Read the model definition and answer for the solid it produces. Units are mm, in the model's axes. Face numbers are marked on the shaded views. A direction names the side the tool comes from. Coordinates: 2 decimals unless noted, no trailing zeros. Loops run counter-clockwise (first coordinate to the right, second up) from the corner with the lowest first, then second, coordinate; pieces in that order, holes last. Notation, with made-up numbers: M 16,74.5 L 35,74.5 A30 ccw 35,101.5 Z; hole C 9.25,64 d11. An arc over 180 degrees is marked long. Put each result on its own line as item: value.
from build123d import *

# Parameters (mm, degrees)
SKETCH1_W            = 150
SKETCH1_H            = 42
BOSS_EXTRUDE1_DEPTH  = 3.2
SKETCH2_W            = 162
SKETCH2_H            = 51
BOSS_EXTRUDE2_DEPTH  = 6
SKETCH3_W            = 6
SKETCH3_H            = 51
BOSS_EXTRUDE3_DEPTH  = 176
BOSS_EXTRUDE4_REACH  = 238.563
SKETCH5_W            = 51
SKETCH5_H            = 6
BOSS_EXTRUDE5_START  = 100
SKETCH1_2_W          = 150
SKETCH1_2_H          = 42
BOSS_EXTRUDE5_DEPTH  = 3.2
SKETCH6_W            = 150
SKETCH6_H            = 6
BOSS_EXTRUDE6_DEPTH  = 70
CUT_EXTRUDE1_REACH   = 142.553
SKETCH7_W            = 9.5
SKETCH7_H            = 39
SKETCH7_R            = 2.75
SKETCH7_3_W          = 6
SKETCH7_3_H          = 39
BOSS_EXTRUDE7_DEPTH  = 54
SKETCH8_W            = 162
SKETCH8_H            = 10
BOSS_EXTRUDE8_DEPTH  = 6
SKETCH9_W            = 150
SKETCH9_H            = 42
CUT_EXTRUDE2_DEPTH   = 3.2
CUT_EXTRUDE3_DEPTH   = 3.2
BOSS_EXTRUDE9_DEPTH  = 6
SKETCH12_W           = 6
SKETCH12_H           = 9.5
BOSS_EXTRUDE10_DEPTH = 6
CUT_EXTRUDE4_REACH   = 235.384
SKETCH13_R           = 4
CUT_EXTRUDE5_REACH   = 202.345
SKETCH14_R           = 1
SKETCH16_W           = 6
SKETCH16_H           = 172
BOSS_EXTRUDE11_DEPTH = 6
BOSS_EXTRUDE15_START = -51
BOSS_EXTRUDE15_DEPTH = 6
SKETCH17_W           = 162
SKETCH17_H           = 63
SKETCH17_W_2         = 150
SKETCH17_H_2         = 56.6
BOSS_EXTRUDE12_DEPTH = 6
SKETCH15_R           = 1
BOSS_EXTRUDE14_DEPTH = 6
FILLET1_R            = 2
FILLET1_OF_MIRROR4_R = 2


with BuildPart() as part:
    # Sketch1 → Boss-Extrude1 (new body)
    with BuildSketch(Plane(origin=(0, 0, 0), x_dir=(1, 0, 0), z_dir=(0, 1, 0))):
        Rectangle(SKETCH1_W, SKETCH1_H)
    extrude(amount=BOSS_EXTRUDE1_DEPTH)

    # Sketch2 → Boss-Extrude2 (add)
    with BuildSketch(Plane.XZ):
        Rectangle(SKETCH2_W, SKETCH2_H)
    extrude(amount=BOSS_EXTRUDE2_DEPTH)

    # Sketch3 → Boss-Extrude3 (add)
    with BuildSketch(Plane(origin=(0, 0, 0), x_dir=(1, 0, 0), z_dir=(0, 1, 0))):
        with Locations((78, 0)):
            Rectangle(SKETCH3_W, SKETCH3_H)
        with Locations((-78, 0)):
            Rectangle(SKETCH3_W, SKETCH3_H)
    extrude(amount=BOSS_EXTRUDE3_DEPTH)

    # Sketch5 → Boss-Extrude4 (add, up to next)
    with BuildSketch(Plane.ZY.offset(-75), mode=Mode.PRIVATE) as boss_extrude4_sk1:
        with Locations((0, 103)):
            Rectangle(SKETCH5_W, SKETCH5_H)
    boss_extrude4_tool1 = extrude(boss_extrude4_sk1.sketch, amount=BOSS_EXTRUDE4_REACH, mode=Mode.PRIVATE) - part.part
    add(boss_extrude4_tool1.solids().sort_by_distance((75, 103, 0))[0])

    # Sketch1<2> → Boss-Extrude5 (add)
    with BuildSketch(Plane(origin=(0, 0, 0), x_dir=(1, 0, 0), z_dir=(0, 1, 0)).offset(BOSS_EXTRUDE5_START)):
        Rectangle(SKETCH1_2_W, SKETCH1_2_H)
    extrude(amount=-BOSS_EXTRUDE5_DEPTH)

    # Sketch6 → Boss-Extrude6 (add)
    with BuildSketch(Plane(origin=(0, 106, 0), x_dir=(1, 0, 0), z_dir=(0, 1, 0))):
        with Locations((0, -22.5)):
            Rectangle(SKETCH6_W, SKETCH6_H)
        with Locations((0, 22.5)):
            Rectangle(SKETCH6_W, SKETCH6_H)
    extrude(amount=BOSS_EXTRUDE6_DEPTH)

    # Sketch7 → Cut-Extrude1 (cut, up to next)
    with BuildSketch(Plane(origin=(0, 106, 0), x_dir=(1, 0, 0), z_dir=(0, 1, 0)), mode=Mode.PRIVATE) as cut_extrude1_sk1:
        with Locations((70.25, 0)):
            Rectangle(SKETCH7_W, SKETCH7_H)
        with Locations((70.25, -14.75)):
            Circle(SKETCH7_R, mode=Mode.SUBTRACT)
        with Locations((70.25, 14.75)):
            Circle(SKETCH7_R, mode=Mode.SUBTRACT)
    cut_extrude1_tool1 = extrude(cut_extrude1_sk1.sketch, amount=-CUT_EXTRUDE1_REACH, mode=Mode.PRIVATE) & part.part
    # Sketch7 → Cut-Extrude1 (cut, up to next)
    with BuildSketch(Plane(origin=(0, 106, 0), x_dir=(1, 0, 0), z_dir=(0, 1, 0)), mode=Mode.PRIVATE) as cut_extrude1_sk2:
        with Locations((70.25, -14.75)):
            Circle(SKETCH7_R)
    cut_extrude1_tool2 = extrude(cut_extrude1_sk2.sketch, amount=-CUT_EXTRUDE1_REACH, mode=Mode.PRIVATE) & part.part
    # Sketch7 → Cut-Extrude1 (cut, up to next)
    with BuildSketch(Plane(origin=(0, 106, 0), x_dir=(1, 0, 0), z_dir=(0, 1, 0)), mode=Mode.PRIVATE) as cut_extrude1_sk3:
        with Locations((70.25, 14.75)):
            Circle(SKETCH7_R)
    cut_extrude1_tool3 = extrude(cut_extrude1_sk3.sketch, amount=-CUT_EXTRUDE1_REACH, mode=Mode.PRIVATE) & part.part
    add(cut_extrude1_tool1.solids().sort_by_distance((70.25, 106, 0))[0], mode=Mode.SUBTRACT)
    add(cut_extrude1_tool2.solids().sort_by_distance((70.25, 106, 14.75))[0], mode=Mode.SUBTRACT)
    add(cut_extrude1_tool3.solids().sort_by_distance((70.25, 106, -14.75))[0], mode=Mode.SUBTRACT)

    # Sketch7<3> → Boss-Extrude7 (add)
    with BuildSketch(Plane(origin=(0, 106, 0), x_dir=(1, 0, 0), z_dir=(0, 1, 0))):
        with Locations((62.5, 0)):
            Rectangle(SKETCH7_3_W, SKETCH7_3_H)
    extrude(amount=BOSS_EXTRUDE7_DEPTH)

    # Sketch8 → Boss-Extrude8 (add)
    with BuildSketch(Plane(origin=(0, 0, -25.5), x_dir=(-1, 0, 0), z_dir=(0, 0, -1))):
        with Locations((0, -1)):
            Rectangle(SKETCH8_W, SKETCH8_H)
    boss_extrude8 = extrude(amount=BOSS_EXTRUDE8_DEPTH)

    # Mirror1: Boss-Extrude8 across plane
    add(boss_extrude8.mirror(Plane.XY))

    # Sketch9 → Cut-Extrude2 (cut)
    with BuildSketch(Plane(origin=(0, 3.2, 0), x_dir=(1, 0, 0), z_dir=(0, 1, 0))):
        Rectangle(SKETCH9_W, SKETCH9_H)
    extrude(amount=-CUT_EXTRUDE2_DEPTH, mode=Mode.SUBTRACT)

    # Sketch10 → Cut-Extrude3 (cut)
    with BuildSketch(Plane.XZ.offset(-96.8)):
        Polygon((-75, -21), (75, -21), (75, -19.5), (65.5, -19.5), (65.5, 19.5), (75, 19.5), (75, 21), (-75, 21), align=None)
    extrude(amount=-CUT_EXTRUDE3_DEPTH, mode=Mode.SUBTRACT)

    # Sketch11 → Boss-Extrude9 (add)
    with BuildSketch(Plane.ZY.offset(-75)):
        Polygon((10, 93.5), (-21, 93.5), (-21, 0), (21, 0), (21, 100), (10, 100), align=None)
    boss_extrude9 = extrude(amount=BOSS_EXTRUDE9_DEPTH)

    # Mirror2: Boss-Extrude9 across plane
    add(boss_extrude9.mirror(Plane(origin=(0, 0, 0), x_dir=(0, 0, 1), z_dir=(1, 0, 0))))

    # Sketch12 → Boss-Extrude10 (add)
    with BuildSketch(Plane(origin=(0, 100, 0), x_dir=(1, 0, 0), z_dir=(0, 1, 0))):
        with Locations((72, -14.75)):
            Rectangle(SKETCH12_W, SKETCH12_H)
    extrude(amount=BOSS_EXTRUDE10_DEPTH)

    # Sketch13 → Cut-Extrude4 (cut, up to next)
    with BuildSketch(Plane.ZY.offset(-69), mode=Mode.PRIVATE) as cut_extrude4_sk1:
        with Locations((0, 20)):
            Circle(SKETCH13_R)
    cut_extrude4_tool1 = extrude(cut_extrude4_sk1.sketch, amount=-CUT_EXTRUDE4_REACH, mode=Mode.PRIVATE) & part.part
    add(cut_extrude4_tool1.solids().sort_by_distance((69, 20, 0))[0], mode=Mode.SUBTRACT)

    # Sketch14 → Cut-Extrude5 (cut, up to next)
    with BuildSketch(Plane.XY.offset(-19.5), mode=Mode.PRIVATE) as cut_extrude5_sk1:
        with Locations((62.5, 103)):
            Circle(SKETCH14_R)
    cut_extrude5_tool1 = extrude(cut_extrude5_sk1.sketch, amount=-CUT_EXTRUDE5_REACH, mode=Mode.PRIVATE) & part.part
    # Sketch14 → Cut-Extrude5 (cut, up to next)
    with BuildSketch(Plane.XY.offset(-19.5), mode=Mode.PRIVATE) as cut_extrude5_sk2:
        with Locations((62.5, 109)):
            Circle(SKETCH14_R)
    cut_extrude5_tool2 = extrude(cut_extrude5_sk2.sketch, amount=-CUT_EXTRUDE5_REACH, mode=Mode.PRIVATE) & part.part
    # Sketch14 → Cut-Extrude5 (cut, up to next)
    with BuildSketch(Plane.XY.offset(-19.5), mode=Mode.PRIVATE) as cut_extrude5_sk3:
        with Locations((62.5, 115)):
            Circle(SKETCH14_R)
    cut_extrude5_tool3 = extrude(cut_extrude5_sk3.sketch, amount=-CUT_EXTRUDE5_REACH, mode=Mode.PRIVATE) & part.part
    add(cut_extrude5_tool1.solids().sort_by_distance((62.5, 103, -19.5))[0], mode=Mode.SUBTRACT)
    add(cut_extrude5_tool2.solids().sort_by_distance((62.5, 109, -19.5))[0], mode=Mode.SUBTRACT)
    add(cut_extrude5_tool3.solids().sort_by_distance((62.5, 115, -19.5))[0], mode=Mode.SUBTRACT)

    # Sketch16 → Boss-Extrude11 (add)
    with BuildSketch(Plane(origin=(0, 0, -25.5), x_dir=(-1, 0, 0), z_dir=(0, 0, -1))):
        with Locations((78, 90)):
            Rectangle(SKETCH16_W, SKETCH16_H)
        with Locations((-78, 90)):
            Rectangle(SKETCH16_W, SKETCH16_H)
    extrude(amount=BOSS_EXTRUDE11_DEPTH)

    # Sketch16<2> → Boss-Extrude15 (add)
    with BuildSketch(Plane(origin=(0, 0, -25.5), x_dir=(-1, 0, 0), z_dir=(0, 0, -1)).offset(BOSS_EXTRUDE15_START)):
        Polygon((75, 100), (75, 4), (81, 4), (81, 176), (75, 176), align=None)
        Polygon((-75, 4), (-75, 100), (-75, 176), (-81, 176), (-81, 4), align=None)
    extrude(amount=-BOSS_EXTRUDE15_DEPTH)

    # Sketch17 → Boss-Extrude12 (add)
    with BuildSketch(Plane.XZ.offset(6)):
        Rectangle(SKETCH17_W, SKETCH17_H)
        Rectangle(SKETCH17_W_2, SKETCH17_H_2, mode=Mode.SUBTRACT)
    extrude(amount=BOSS_EXTRUDE12_DEPTH)

    # Sketch15 → Boss-Extrude14 (add)
    with BuildSketch(Plane(origin=(0, 0, -25.5), x_dir=(-1, 0, 0), z_dir=(0, 0, -1))):
        with BuildLine():
            ThreePointArc((-62.5, 121), (-51.27502784, 113.242640687), (-54.562746067, 100))
            Line((-54.562746067, 100), (-46.5, 100))
            Line((-46.5, 100), (-46.5, 121))
            Line((-46.5, 121), (-62.5, 121))
        make_face()
        with BuildLine():
            ThreePointArc((-62.5, 121), (-73.72497216, 113.242640687), (-70.437253933, 100))
            Line((-70.437253933, 100), (-54.562746067, 100))
            ThreePointArc((-54.562746067, 100), (-51.27502784, 113.242640687), (-62.5, 121))
        make_face()
        with Locations(Location((-62.5, 103, 0), (0, 0, 180))):
            Circle(SKETCH15_R, mode=Mode.SUBTRACT)
        with Locations(Location((-62.5, 109, 0), (0, 0, 180))):
            Circle(SKETCH15_R, mode=Mode.SUBTRACT)
        with Locations(Location((-62.5, 115, 0), (0, 0, 180))):
            Circle(SKETCH15_R, mode=Mode.SUBTRACT)
    boss_extrude14 = extrude(amount=BOSS_EXTRUDE14_DEPTH)

    # Fillet1
    fillet1_edges = [part.edges().sort_by_distance(p)[0] for p in [
        (46.5, 121, -28.5),
        (46.5, 100, -28.5),
    ]]
    fillet(fillet1_edges, radius=FILLET1_R)

    # Mirror4: Boss-Extrude14 across plane
    add(boss_extrude14.mirror(Plane.XY))

    # Fillet1 of Mirror4
    fillet1_of_mirror4_edges = [part.edges().sort_by_distance(p)[0] for p in [
        (46.5, 121, 28.5),
        (46.5, 100, 28.5),
    ]]
    fillet(fillet1_of_mirror4_edges, radius=FILLET1_OF_MIRROR4_R)


solid = part.part
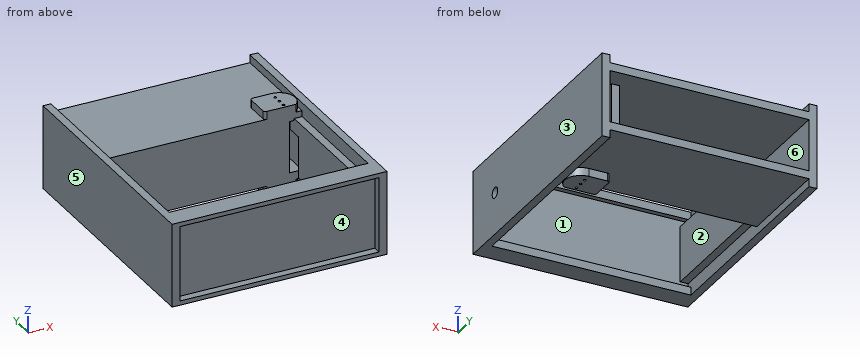
1) Find section B-B, the plane y = 20. Write down the section's boundary in (x, z).
Answer list:
outline: M -81,-31.5 L -75,-31.5 L -75,-21 L -69,-21 L -69,21 L -75,21 L -75,31.5 L -81,31.5 Z; M 69,-21 L 75,-21 L 75,-31.5 L 81,-31.5 L 81,-4 L 69,-4 Z; M 69,4 L 81,4 L 81,31.5 L 75,31.5 L 75,21 L 69,21 Z
2) Find section D-D, the plane x = -5. Write down the section's boundary in (y, z), plus the area to 3 significant figures.
Answer list:
outline: M -12,-31.5 L 4,-31.5 L 4,-25.5 L 0,-25.5 L 0,25.5 L 4,25.5 L 4,31.5 L -12,31.5 L -12,28.3 L -6,28.3 L -6,-28.3 L -12,-28.3 Z; M 100,-25.5 L 176,-25.5 L 176,-19.5 L 106,-19.5 L 106,19.5 L 176,19.5 L 176,25.5 L 100,25.5 Z
area: 1,610 mm^2
3) Given pin 1 Ø3 at (x, z) = (71.5, -1.5) entering from +Y; pin 2 Ø1.8 at (x, y) = (-71, 96.5) entering from -Z; pin 3 Ø1.2 at (x, y) = (62.5, 109) entering from -Z; pin 4 Ø1.6 at (x, y) = (62.5, 103.5) entering from -Z, each flat-ended and moving along its own axis, determine where each tip first touches the part or whether it passes through.
Answer list:
pin 1: stops at y = 93.5
pin 2: stops at z = 10
pin 3: stops at z = -19.5
pin 4: stops at z = -31.5
4) Find section A-A, the plane z = 0. Write down the section's boundary in (x, y), plus the area to 3 significant figures.
Answer list:
outline: M -81,-12 L -75,-12 L -75,-6 L 75,-6 L 75,-12 L 81,-12 L 81,16 L 69,16 L 69,0 L -69,0 L -69,93.5 L -75,93.5 L -75,100 L 65.5,100 L 65.5,160 L 59.5,160 L 59.5,106 L -75,106 L -75,176 L -81,176 Z; M 69,24 L 81,24 L 81,176 L 75,176 L 75,93.5 L 69,93.5 Z
area: 5,350 mm^2
5) Straight lines are drawn through the part: line 1 (Y direction, x = 62.5, z = -23.5); line 2 (X direction, y = 109, z = 29.05); line 3 (Y direction, x = 62.5, z = 27.35). For each, find the intervals that lie inside material, in ascending order. Write a range as [from, to].
Answer list:
line 1: y = [-6, 0], [100, 102], [104, 108], [110, 114], [116, 176]
line 2: x = [-81, -75], [46.5, 61.5], [63.5, 74.5], [75, 81]
line 3: y = [-6, 4], [100, 102], [104, 108], [110, 114], [116, 121]
6) Determine the mould class of the marked faces 1, 2, 3 and 4 for opening direction Y: released by +Y, released by -Y, zero draft, split by the parting line, or undercut.
Answer list:
face 1: undercut
face 2: undercut
face 3: zero draft
face 4: released by -Y
7) Which of the six approach directions +Z, -Z, +X, -X, +Y, -Y give full straight-line access (tool end or side, diameter ignored) to the marked faces 5 and 6?
Answer list:
face 5: +Z, -Z, -X, +Y, -Y
face 6: +Y
8) Find section C-C, the plane y = 85. Write down the section's boundary in (x, z), plus the area to 3 significant figures.
Answer list:
outline: M -81,-31.5 L -75,-31.5 L -75,-21 L -69,-21 L -69,21 L -75,21 L -75,31.5 L -81,31.5 Z; M 69,-21 L 75,-21 L 75,-31.5 L 81,-31.5 L 81,31.5 L 75,31.5 L 75,21 L 69,21 Z
area: 1,260 mm^2
